from build123d import *

# Parameters (mm, degrees)
SKETCH1_R           = 22.5
BOSS_EXTRUDE1_DEPTH = 2.5
SKETCH2_R           = 6
BOSS_EXTRUDE2_DEPTH = 2
CUT_EXTRUDE1_DEPTH  = 10


with BuildPart() as part:
    # Sketch1 → Boss-Extrude1 (new body)
    with BuildSketch(Plane.XY):
        Circle(SKETCH1_R)
    extrude(amount=BOSS_EXTRUDE1_DEPTH)

    # Sketch2 → Boss-Extrude2 (add)
    with BuildSketch(Plane.XY.offset(2.5)):
        Circle(SKETCH2_R)
    extrude(amount=BOSS_EXTRUDE2_DEPTH)

    # Sketch3 → Cut-Extrude1 (cut)
    with BuildSketch(Plane.XY.offset(4.5)):
        Polygon((-4, 2), (-4, -2), (4, -2), (4, 2), (1, 2), (1, 4), (-1, 4), (-1, 2), align=None)
    extrude(amount=-CUT_EXTRUDE1_DEPTH, mode=Mode.SUBTRACT)


solid = part.part
Read the model definition and answer for the solid it produces. Units are mm, in the model's axes. A direction names the side the tool comes from. Round coordinates to 2 decimals unless told otherwise and drop trailing zeros. Order: outer loops, then holes, each group sorted by start corner. A loop starts at its lowest first (then second) coordinate and runs counter-clockwise, first axis right, second up.
1) For faces 1 (the face through (5, -5, 2.5)), 2 (the face through (0, -2, 2)), 3 (the face through (0, -5, 0)), determine the directions among +Z, -Z, +X, -X, +Y, -Y from which every point of the face is accessible in a straight line to the end or side of a thin tool.
2) The part is cut by section C-C on z = 1.85. Write down the section's boundary in (x, y).
3) Straight lines are drawn through the part: L1, parallel to Z at x = 19, y = 4.5; L2, parallel to Y at x = 2, z = 3.55; L3, parallel to Y at x = 2.5, z = 4.35. For each, find the intervals that lie inside material, in ascending order.
4) The part is cut by section D-D on x = 18. Write down the section's boundary in (y, z).
5) The part is cut by section A-A on x = 0. Write down the section's boundary in (y, z).
6) Flat-ended cylindrical pins translate along their axes: pin 1 (5 mm diameter, centred on x = 16, y = 10.5, fed in from -Z); pin 2 (1.6 mm diameter, centred on y = 3, z = 3.5, fed in from -X); pin 3 (1.6 mm diameter, centred on x = -0.5, z = 2.5, fed in from -Y); pin 4 (2.5 mm diameter, centred on x = -3, z = 1.5, fed in from -Y). Find the tip coordinate at first contact, or state that the pin passes through.
7) The part is cut by section B-B on y = 0. Write down the section's boundary in (x, z).
Resolved:
1. face 1: +Z
1. face 2: +Z, -Z
1. face 3: -Z, +X, -X, +Y, -Y
2. outline: circle Ø45 at (0, 0); hole (-4, -2) - (4, -2) - (4, 2) - (1, 2) - (1, 4) - (-1, 4) - (-1, 2) - (-4, 2) - close
3. L1: z = 0 to 2.5
3. L2: y = -5.66 to -2, 2 to 5.66
3. L3: y = -5.45 to -2, 2 to 5.45
4. outline: (-13.5, 0) - (13.5, 0) - (13.5, 2.5) - (-13.5, 2.5) - close
5. outline: (-22.5, 0) - (-2, 0) - (-2, 4.5) - (-6, 4.5) - (-6, 2.5) - (-22.5, 2.5) - close; (4, 0) - (22.5, 0) - (22.5, 2.5) - (6, 2.5) - (6, 4.5) - (4, 4.5) - close
6. pin 1: stops at z = 0
6. pin 2: stops at x = -5.58
6. pin 3: stops at y = -22.5
6. pin 4: stops at y = -22.43
7. outline: (-22.5, 0) - (-4, 0) - (-4, 4.5) - (-6, 4.5) - (-6, 2.5) - (-22.5, 2.5) - close; (4, 0) - (22.5, 0) - (22.5, 2.5) - (6, 2.5) - (6, 4.5) - (4, 4.5) - close
